Build history of the part. All positions in model axes, mm. Face numbers are marked on the shaded views. Round coordinates to 2 decimals unless told otherwise and drop trailing zeros. Write each loop counter-clockwise with the first axis right and the second up, starting at its lowest first coordinate (ties: lowest second). Pieces come first, ordered by that corner, then holes. Notation, with made-up numbers: (6.5, 64.25) -> (24.5, 64.25) arc R11 cw to (24.5, 73.25) -> close; hole circle Ø2 at (-29.75, -34). An arc over 180 degrees is marked (long way). One line per question, with ' | ' between items.
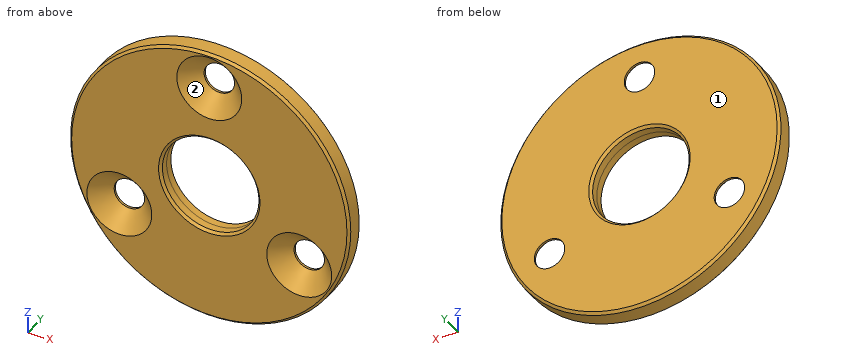
from build123d import *

# Parameters (mm, degrees)
F0_R           = 29
F0_R_2         = 10
F1_DEPTH       = 2
F1_DEPTH_BACK  = 2
F3_D           = 6.3
F3_CSINK_D     = 13.44
F3_CSINK_ANGLE = 90
F4_SIZE        = 0.5


with BuildPart() as f1:
    # F0 (on Front) → F1 (new body, two sides)
    with BuildSketch(Plane.XZ) as f1_sk:
        Circle(F0_R)
        Circle(F0_R_2, mode=Mode.SUBTRACT)
    extrude(amount=F1_DEPTH)
    extrude(f1_sk.sketch, amount=-F1_DEPTH_BACK)

    # F3 (through all)
    with Locations(Plane.XZ.offset(2)):
        with Locations((0, 21.5), (-18.6195461814, -10.75), (18.6195461814, -10.75)):
            CounterSinkHole(F3_D / 2, F3_CSINK_D / 2, counter_sink_angle=F3_CSINK_ANGLE)

    # F4
    f4_edges = [f1.edges().sort_by_distance(p)[0] for p in [
        (-29, -2, 0),
        (29, -1, 0),
        (-29, 0, 0),
        (-10, 2, 0),
        (-10, -2, 0),
    ]]
    chamfer(f4_edges, length=F4_SIZE)


solid = f1.part
(1) Slice it at A-A (z = 0). Write the cut outline in (x, y), then the cut area to 3 significant figures.
Calculated:
outline: (-29, -1.5) -> (-28.5, -2) -> (-10.5, -2) -> (-10, -1.5) -> (-10, 1.5) -> (-10.5, 2) -> (-28.5, 2) -> (-29, 1.5) -> close; (10, -1.5) -> (10.5, -2) -> (28.5, -2) -> (29, -1.5) -> (29, 1.5) -> (28.5, 2) -> (10.5, 2) -> (10, 1.5) -> close | area: 151 mm2
(2) Slice it at D-D (z = -13). State how many separate pieces and enclosed holes the cut face has, then the cut area to 3 significant figures.
Calculated:
separate pieces: 3 | enclosed holes: 0 | area: 141 mm2
(3) Wall check: line 1 (X direction, y = 0.3, z = -14.5); line 2 (Z direction, x = 0, y = -0.35); line 3 (X direction, y = -1.55, z = -7). Give the ranges that are in metal, low to high. Write a range as from..to.
Calculated:
line 1: -25.11..-20.96, -16.28..16.28, 20.96..25.11 | line 2: -29..-10, 10..16.43, 26.57..29 | line 3: -28.09..-23.64, -13.59..-7.21, 7.21..13.59, 23.64..28.09
(4) Drop flat-ended pins along their axis: pin 1 (2 mm diameter, centred on y = 1, z = 17, fed in from -X); pin 2 (8 mm diameter, centred on x = 18.62, z = -10.75, fed in from -Y); pin 3 (1.5 mm diameter, centred on y = 0, z = -11, fed in from -X). Give the stop position or say it passes through.
Calculated:
pin 1: x = -24.19 | pin 2: y = 0.72 | pin 3: x = -27.13
(5) Mould opens along X. For the marked faces 1 and 2 say: pulls with the +X half, pulls with the -X half, needs draft (parallel to the pull), parting line crosses it, or undercut.
Calculated:
face 1: needs draft | face 2: undercut
(6) Slice it at C-C (y = 0.6). Write the cut outline in (x, z).
Calculated:
outline: circle Ø58 at (0, 0); hole circle Ø8.24 at (-18.62, -10.75); hole circle Ø20 at (0, 0); hole circle Ø8.24 at (0, 21.5); hole circle Ø8.24 at (18.62, -10.75)
(7) Slice it at B-B (x = 0). Write the cut outline in (y, z).
Calculated:
outline: (-2, -28.5) -> (-1.5, -29) -> (1.5, -29) -> (2, -28.5) -> (2, -10.5) -> (1.5, -10) -> (-1.5, -10) -> (-2, -10.5) -> close; (-2, 10.5) -> (-1.5, 10) -> (1.5, 10) -> (2, 10.5) -> (2, 18.35) -> (1.57, 18.35) -> (-2, 14.78) -> close; (-2, 28.22) -> (1.57, 24.65) -> (2, 24.65) -> (2, 28.5) -> (1.5, 29) -> (-1.5, 29) -> (-2, 28.5) -> close
